Autodesk Inventor part; units mm, degrees
ref_plane "YZ Plane" through (0, 0, 0) normal (1, 0, 0) x (0, 1, 0)
ref_plane "XZ Plane" through (0, 0, 0) normal (0, 1, 0) x (-1, 0, 0)
ref_plane "XY Plane" through (0, 0, 0) normal (0, 0, 1) x (1, 0, 0)
sketch "Sketch1" plane through (0, 0, 0) normal (0, 0, 1) x (1, 0, 0)
  arc A0 (0.8988, -14.2961) -> (0.8988, 14.2961) centre (0, 0) ccw construction
  arc A1 (-150.7006, 23.8269) -> (-150.7006, -23.8269) centre (-152.1985, 0) ccw construction
  line L0 (0.8988, -14.2961) -> (-150.7006, -23.8269) construction
  line L1 (0.8988, 14.2961) -> (-150.7006, 23.8269) construction
  dimension "Belt_Teeth" = 85
  dimension "Belt_Pitch2" = 5
  dimension "d0" = 28.6487
  dimension "d1" = 47.7479
  dimension "d2" = 43.2026
  dimension "d3" = 78.0001
  dimension "Center_Distance" = 152.1985
  dimension "d5" = 151.8987
sketch "Sketch2" plane through (0, 0, 0) normal (0, 0, 1) x (1, 0, 0)
  line L0 (35.7235, 34.2567) -> (40.7235, 34.2567)
  point P0 (0, 0)
  dimension "Belt_Pitch2" = 5
sketch "Sketch4" plane through (0, 0, 0) normal (0, 0, 1) x (1, 0, 0)
  line L0 (-16.1422, -21.869) -> (-14.1422, -21.869)
  line L1 (-16.1422, -21.869) -> (-16.1422, -20.349)
  arc A0 (-15.5872, -20.904) -> (-16.1422, -20.349) centre (-16.1422, -20.904) ccw
  line L2 (-15.5872, -20.904) -> (-15.5872, -20.959)
  arc A1 (-15.5872, -20.959) -> (-15.4372, -21.109) centre (-15.4372, -20.959) ccw
  line L3 (-15.4372, -21.109) -> (-14.8472, -21.109)
  line L4 (-14.1422, -21.869) -> (-14.1422, -20.349)
  arc A2 (-14.1422, -20.349) -> (-14.6972, -20.904) centre (-14.1422, -20.904) ccw
  arc A3 (-14.8472, -21.109) -> (-14.6972, -20.959) centre (-14.8472, -20.959) ccw
  line L5 (-14.6972, -20.959) -> (-14.6972, -20.904)
  line L6 (0.8988, 14.2961) -> (-150.7006, 23.8269) construction
  arc A4 (-150.7006, 23.8269) -> (-150.7006, -23.8269) centre (-152.1985, 0) ccw construction
  line L7 (0.8988, -14.2961) -> (-150.7006, -23.8269) construction
  arc A5 (0.8988, -14.2961) -> (0.8988, 14.2961) centre (0, 0) ccw construction
  arc A6 (-150.6378, 24.8249) -> (-150.6378, -24.8249) centre (-152.1985, 0) ccw
  line L8 (-150.6378, 24.8249) -> (0.9615, 15.2942)
  arc A7 (0.9615, -15.2942) -> (0.9615, 15.2942) centre (0, 0) ccw
  line L9 (0.9615, -15.2942) -> (-150.6378, -24.8249)
  arc A8 (-150.7633, 22.8289) -> (-150.7633, -22.8289) centre (-152.1985, 0) ccw
  line L10 (-150.7633, 22.8289) -> (0.836, 13.2981)
  arc A9 (0.836, -13.2981) -> (0.836, 13.2981) centre (0, 0) ccw
  line L11 (0.836, -13.2981) -> (-150.7633, -22.8289)
  point P0 (-15.1422, -21.109)
  point P1 (-15.1422, -21.869)
  dimension "d9" = 2
  dimension "d10" = 1.52
  dimension "d11" = 0.76
  dimension "d12" = 0.555
  dimension "d13" = 0.555
  dimension "d14" = 0.15
  dimension "d15" = 0.15
  dimension "belt_thickness" = 2
  dimension "d44" = 1
extrude "Extrusion2" add sketch "Sketch4" along normal mid plane 8.5 contours L8 A7 L9 A6
sketch "Sketch5" plane through (0, 0, 4.25) normal (0, 0, 1) x (1, 0, 0)
  line L0 (-150.7633, 22.8289) -> (0.836, 13.2981) construction
  arc A0 (0.836, -13.2981) -> (0.836, 13.2981) centre (0, 0) ccw construction
  line L1 (0.836, -13.2981) -> (-150.7633, -22.8289) construction
  arc A1 (-150.7633, 22.8289) -> (-150.7633, -22.8289) centre (-152.1985, 0) ccw construction
  arc A2 (-150.6378, 24.8249) -> (-150.6378, -24.8249) centre (-152.1985, 0) ccw construction
  line L2 (-150.6378, -24.8249) -> (0.9615, -15.2942) construction
  arc A3 (0.9615, -15.2942) -> (0.9615, 15.2942) centre (0, 0) ccw construction
  line L3 (0.9615, 15.2942) -> (-150.6378, 24.8249) construction
  line L4 (-7.7556, -2.6989) -> (-5.7556, -2.6989)
  line L5 (-7.7556, -2.6989) -> (-7.7556, -1.1789) construction
  arc A4 (-7.2006, -1.7339) -> (-7.7556, -1.1789) centre (-7.7556, -1.7339) ccw
  line L6 (-7.2006, -1.7339) -> (-7.2006, -1.7889)
  arc A5 (-7.2006, -1.7889) -> (-7.0506, -1.9389) centre (-7.0506, -1.7889) ccw
  line L7 (-7.0506, -1.9389) -> (-6.4606, -1.9389)
  line L8 (-5.7556, -2.6989) -> (-5.7556, -1.1789)
  arc A6 (-5.7556, -1.1789) -> (-6.3106, -1.7339) centre (-5.7556, -1.7339) ccw
  arc A7 (-6.4606, -1.9389) -> (-6.3106, -1.7889) centre (-6.4606, -1.7889) ccw
  line L9 (-6.3106, -1.7889) -> (-6.3106, -1.7339)
  line L10 (-8.3106, -1.7339) -> (-8.3106, -1.7889)
  arc A8 (-7.7556, -1.1789) -> (-8.3106, -1.7339) centre (-7.7556, -1.7339) ccw
  arc A9 (-8.4606, -1.9389) -> (-8.3106, -1.7889) centre (-8.4606, -1.7889) ccw
  line L11 (-8.4606, -1.9389) -> (-9.0506, -1.9389)
  line L12 (-7.7556, -2.6989) -> (-9.7556, -2.6989)
  line L13 (-9.2006, -1.7889) -> (-9.2006, -1.7339)
  arc A10 (-9.2006, -1.7339) -> (-9.7556, -1.1789) centre (-9.7556, -1.7339) ccw
  line L14 (-9.7556, -2.6989) -> (-9.7556, -1.1789)
  arc A11 (-9.2006, -1.7889) -> (-9.0506, -1.9389) centre (-9.0506, -1.7889) ccw
  line L15 (-17.66, -0.8495) -> (-14.922, -0.8495) construction
  line L16 (-14.922, -0.8495) -> (-14.922, -2.3671) construction
  line L17 (-14.922, -2.3671) -> (-17.66, -2.3671) construction
  line L18 (-17.66, -2.3671) -> (-17.66, -0.8495) construction
  arc A12 (-15.6383, -1.7102) -> (-16.7483, -1.7102) centre (-16.1933, -1.7102) ccw construction
  line L19 (-16.7483, -1.7102) -> (-16.7483, -1.7652) construction
  arc A13 (-16.8983, -1.9152) -> (-16.7483, -1.7652) centre (-16.8983, -1.7652) ccw construction
  line L20 (-16.7483, -1.7102) -> (-16.7483, -1.9152) construction
  line L21 (-15.6383, -1.7102) -> (-15.6383, -1.9152) construction
  point P0 (-6.7556, -1.9389)
  point P1 (-6.7556, -2.6989)
  point P2 (-8.7556, -2.6989)
  point P3 (-8.7556, -1.9389)
  dimension "d22" = 2
  dimension "d23" = 1.52
  dimension "d24" = 0.76
  dimension "d25" = 0.555
  dimension "d26" = 0.555
  dimension "d27" = 0.15
  dimension "d28" = 0.15
  dimension "d29" = 0.76
  dimension "d30" = 1
  dimension "d31" = 2
  dimension "d32" = 0.59
  dimension "d34" = 0.555
  dimension "d35" = 0
  dimension "d36" = 0
  dimension "d37" = 0.15
  dimension "d38" = 0.055
  dimension "d39" = 0.055
  dimension "d40" = 0
  dimension "d41" = 0
  dimension "d42" = 0.205
  dimension "d43" = 0.205
equation "\"d13\" = d12"
equation "\"d15\" = d14"
equation "\"d44\" = 0.5 * belt_thickness"
equation "\"d26\" = d25"
equation "\"d28\" = d27"
equation "\"d31\" = d22"
equation "\"d43\" = d42"
equation "\"Belt_Teeth\" = 85"
equation "\"Belt_Pitch\" = 3"
equation "\"HTD_5mm\" = 5"
equation "\"GT2_3mm\" = 3"
equation "\"Center_Distance_Copy\" = Center_Distance"
properties part number "GP6-014 - 85T belt" material "Rubber"
Input: part model. Units: mm. Frame: model coordinates. A direction names the side the tool comes from. Give positions to 0.01 mm unless a question says otherwise; leave off trailing zeros. Order: outer loops, then holes, each group sorted by start corner. A loop starts at its lowest first (then second) coordinate and runs counter-clockwise, first axis right, second up. Notation, with made-up numbers: (51, 8.5) - (94, 8.5) arc R6 cw to (94, 18.5) - close; hole circle Ø9 at (-13, 82). An arc over 180 degrees is marked (long way). Answer as a JSON object with one key per item and string values. Group by question number.
Q1. Cut plane B-B, the plane z = 0.25. Output: boundary loops of the cut face in (x, y), then the cut area to 3 significant figures.
Q2. Set-up query: faces 1 (the face through (-76.02, 18.13, -0.06)), 2 (the face through (-81, 19, 4.25)). Return all of +Z, -Z, +X, -X, +Y, -Y with unobstructed straight access to the full face (end or side cutting, diameter ignored); none if empty.
Q3. Line query: probe 1 along X at (y, z) = (0.5, 2.25); probe 2 along Y at (x, z) = (0.5, 3.25); probe 3 along Y at (x, z) = (-80, -0.5). Output: solid intervals per line, ascending.
Q4. Cut plane A-A, the plane y = 0. Output: boundary loops of the cut face in (x, z), then the cut area to 3 significant figures.
Q5. Cut plane C-C, the plane x = -110. Output: boundary loops of the cut face in (y, z), then the cut area to 3 significant figures.
Q6. First-contact query: pin 1 Ø12 at (x, y) = (-102.5, -13) entering from -Z; pin 2 Ø5 at (y, z) = (-13, 0.5) entering from +X; pin 3 Ø4 at (x, z) = (-122, 0.5) entering from +Y; pin 4 Ø3 at (y, z) = (-1.5, -2.5) entering from -X. Flat tips, straight axial feed; report the tip coordinate or a pass-through.
Q7. Mould query, pull axis X, two halves, no side actions, for faces 3 (the face through (-81, 19, -4.25)), 4 (the face through (-73.777, -19.993, -0.059)), 5 (the face through (-73.902, -17.997, -0.059)), 6 (the face through (13.32, 0.28, -0.06)). Classes: pulls with the +X half, pulls with the -X half, needs draft (parallel to the pull), parting line crosses it, or undercut.
Results:
{
 "1": {"outline": "(-150.64, -24.82) - (0.96, -15.29) arc R15.32 ccw to (0.96, 15.29) - (-150.64, 24.82) arc R24.87 ccw (long way) to start; hole (-150.76, -22.83) - (0.84, -13.3) arc R13.32 ccw to (0.84, 13.3) - (-150.76, 22.83) arc R22.87 ccw (long way) to start", "area": "850 mm^2"},
 "2": {"face 1": "+Z, -Z", "face 2": "+Z, +X, -X, +Y, -Y"},
 "3": {"probe 1": "-177.07 to -175.07, 13.31 to 15.32", "probe 2": "-15.32 to -13.32, 13.32 to 15.32", "probe 3": "-20.38 to -18.38, 18.38 to 20.38"},
 "4": {"outline": "(-177.07, -4.25) - (-175.07, -4.25) - (-175.07, 4.25) - (-177.07, 4.25) - close; (13.32, -4.25) - (15.32, -4.25) - (15.32, 4.25) - (13.32, 4.25) - close", "area": "34.0 mm^2"},
 "5": {"outline": "(-22.27, -4.25) - (-20.27, -4.25) - (-20.27, 4.25) - (-22.27, 4.25) - close; (20.27, -4.25) - (22.27, -4.25) - (22.27, 4.25) - (20.27, 4.25) - close", "area": "34.1 mm^2"},
 "6": {"pin 1": "through", "pin 2": "x = 11.16", "pin 3": "y = 23.15", "pin 4": "x = -177.07"},
 "7": {"face 3": "needs draft", "face 4": "pulls with the +X half", "face 5": "undercut", "face 6": "undercut"}
}
